Print and shaded views of the part. All mm, measured from the part's lowest x, y and z. A direction names the side the tool comes from. Round coordinates to 2 decimals unless told otherwise and drop trailing zeros. Loops run counter-clockwise (first coordinate to the right, second up) from the corner with the lowest first, then second, coordinate; pieces in that order, holes last. Notation, with made-up numbers: (51.25, 65) - (80.25, 65) arc R36 cw to (80.25, 102) - close; hole circle Ø9 at (33, 57.25). An arc over 180 degrees is marked (long way). Put each result on its own line as item: value. Start each with the question number.
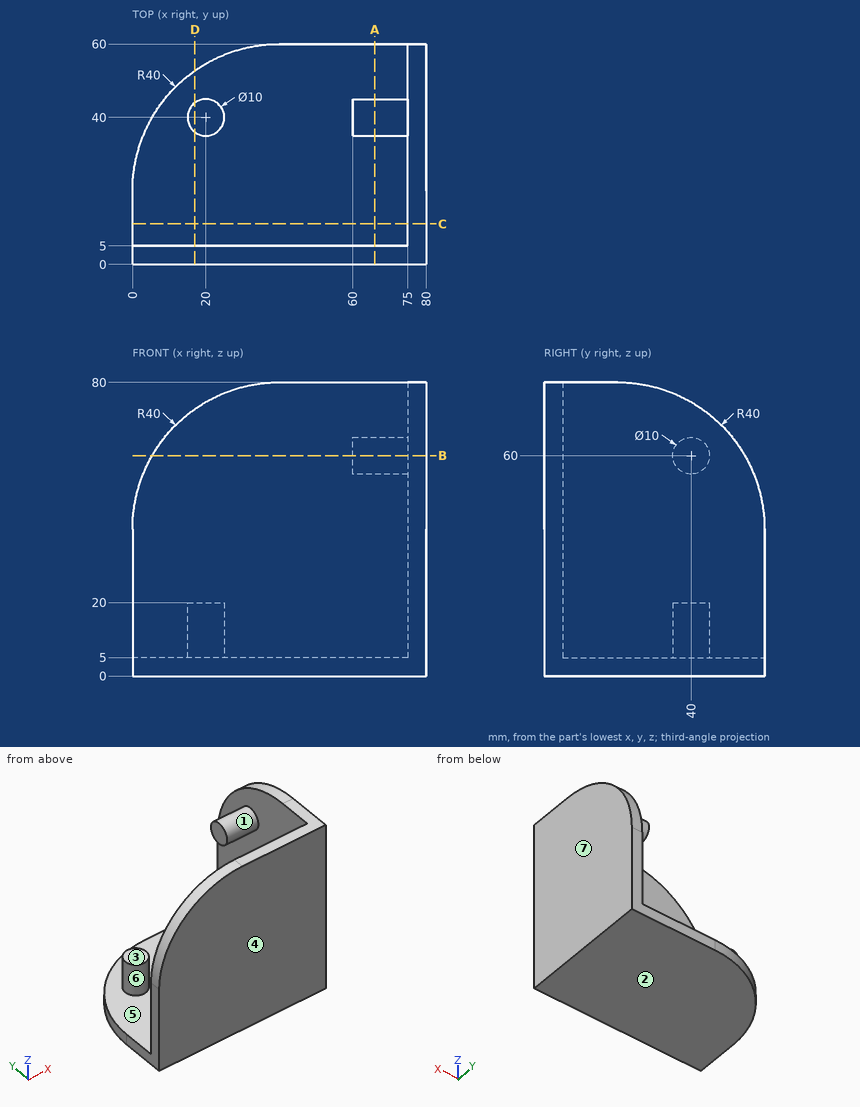
Item 1: Slice it at C-C (y = 11). Give the cut face in (x, z).
Item 2: Drop flat-ended pins along their axis: pin 1 Ø8 at (y, z) = (8, 14) entering from -X; pin 2 Ø1.5 at (x, z) = (47, 47) entering from +Y; pin 3 Ø5 at (y, z) = (41.5, 61) entering from -X; pin 4 Ø2 at (x, y) = (13.5, 16) entering from +Z. Give the stop position or say it passes through.
Item 3: Drill centre lines: probe 1 along Y at (x, z) = (47, 42); probe 2 along X at (y, z) = (55, 41.5). Where is each one in solid material? Low to high. Write a range as [from, to].
Item 4: Which spindle directions (+Z, -Z, +X, -X, +Y, -Y) get a long thin tool onto all of the face, cutting with end or side? Do the marked faces 1, 2 and 3. Say none if no direction does.
Item 5: Slice it at B-B (z = 60). Give the cut face in (x, y), plus the area to 3 significant figures.
Item 6: Slice it at D-D (x = 17). Give the cut face in (y, z), plus the area to 3 significant figures.
Item 7: Slice it at A-A (x = 66). Give the cut face in (y, z).
Item 8: Two-plate mould, pull along X, no slides. Class the marked faces 4, 5, 6 and 7: pulls with the +X half, pulls with the -X half, needs draft (parallel to the pull), parting line crosses it, or undercut.
Computed values:
1. outline: (0, 0) - (80, 0) - (80, 80) - (75, 80) - (75, 5) - (0, 5) - close
2. pin 1: stops at x = 0
2. pin 2: stops at y = 5
2. pin 3: stops at x = 60
2. pin 4: stops at z = 5
3. probe 1: y = [0, 5]
3. probe 2: x = [75, 80]
4. face 1: -X
4. face 2: -Z, +X, -X, +Y, -Y
4. face 3: +Z, -X, +Y
5. outline: (5.36, 0) - (80, 0) - (80, 54.64) - (75, 54.64) - (75, 45) - (60, 45) - (60, 35) - (75, 35) - (75, 5) - (5.36, 5) - close
5. area: 771 mm^2
6. outline: (0, 0) - (52.73, 0) - (52.73, 5) - (44, 5) - (44, 20) - (36, 20) - (36, 5) - (5, 5) - (5, 72.73) - (0, 72.73) - close
6. area: 722 mm^2
7. outline: (0, 0) - (60, 0) - (60, 5) - (5, 5) - (5, 80) - (0, 80) - close; circle Ø10 at (40, 60)
8. face 4: needs draft
8. face 5: undercut
8. face 6: undercut
8. face 7: pulls with the +X half
